Check sheet for the modelled part. Datum: model origin and axes. Units: mm. Give positions to 0.01 mm unless a question says otherwise; leave off trailing zeros. Order: outer loops, then holes, each group sorted by start corner. A loop starts at its lowest first (then second) coordinate and runs counter-clockwise, first axis right, second up.
Autodesk Fusion 360 part; units mm, degrees
sketch "Esquisse1" plane through (0, 0, 0) normal (0, 0, 1) x (1, 0, 0)
  circle A0 centre (0, 0) radius 4
  circle A1 centre (0, 0) radius 3
  dimension "d1" = 8
  dimension "d2" = 6
extrude "Extrusion1" add sketch "Esquisse1" along normal blind 140
hole "Perçage1" at (0, 0, 0) direction (0, 1, 0) diameter 3.5 depth 8 tip angle 180
hole "Perçage2" at (0, 4, 96) direction (0, -1, 0) diameter 3.5 depth 8 tip angle 180
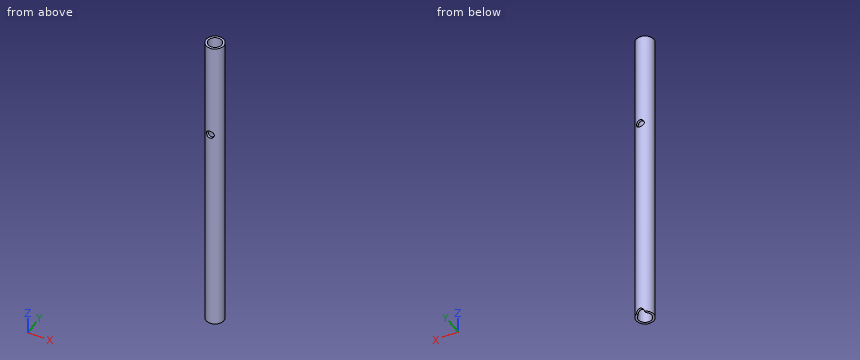
(1) Cross-section at C-C on z = 67.5. Enter the section's corners in (x, y), then the cut area to 3 significant figures.
Response values:
outline: circle Ø8 at (0, 0); hole circle Ø6 at (0, 0)
area: 22.0 mm2
(2) Gauge pin test, flat ends, axial feed: pin 1 Ø1.5 at (y, z) = (1, 36.5) entering from +X; pin 2 Ø1 at (x, z) = (-1.5, 109.5) entering from +Y. Record the tip position at first contact, or that the pin passes through.
Response values:
pin 1: stops at x = 3.99
pin 2: stops at y = 3.87
(3) Material ranges on L1, parallel to X at y = 0.25, z = 53; L2, parallel to Z at x = 0, y = -3.6; L3, parallel to Y at x = 0, z = 33, recorded low to high.
Response values:
L1: x = -3.99 to -2.99, 2.99 to 3.99
L2: z = 0 to 94.25, 97.75 to 140
L3: y = -4 to -3, 3 to 4
(4) Cross-section at A-A on x = 0. Enter the section's corners in (y, z), then the cut area to 3 significant figures.
Response values:
outline: (-4, 0) - (-3, 0) - (-3, 94.25) - (-4, 94.25) - close; (-4, 97.75) - (-3, 97.75) - (-3, 140) - (-4, 140) - close; (3, 1.75) - (4, 1.75) - (4, 94.25) - (3, 94.25) - close; (3, 97.75) - (4, 97.75) - (4, 140) - (3, 140) - close
area: 271 mm2
(5) Cross-section at B-B on y = 0. Enter the section's corners in (x, z).
Response values:
outline: (-4, 0) - (-3, 0) - (-3, 140) - (-4, 140) - close; (3, 0) - (4, 0) - (4, 140) - (3, 140) - close
